Could you check a few things on this drawing? It's one solid part, dimensions in mm from its lowest x, y, z. A direction names the side the tool comes from. Round coordinates to 2 decimals unless told otherwise and drop trailing zeros. Write each loop counter-clockwise with the first axis right and the second up, starting at its lowest first coordinate (ties: lowest second). Pieces come first, ordered by that corner, then holes. Notation, with made-up numbers: (-38.5, 60.5) - (-17.5, 60.5) arc R3 cw to (-17.5, 65.5) - close; hole circle Ø4 at (-35.75, 81). An arc over 180 degrees is marked (long way). Use one line per item in the form item = value. Start each with the question number.
1. I want a section at C-C, the plane z = 17.5. List the corners of the cut face in (x, y) for me.
2. I want a section at B-B, the plane x = 5. List the corners of the cut face in (y, z) for me, plus the area to 3 significant figures.
3. Which directions (+Z, -Z, +X, -X, +Y, -Y) give clear straight access to the entire face, cutting with the end or side of a thin tool? Please do the marked faces 5, 6, 7 and 8.
4. If I drill on line 1 along X through (y, z) = (8.75, 17); line 2 along Y through (x, z) = (1.5, 9); line 3 along X through (y, z) = (17.5, 19), over which ranges is the centre line in solid material (lowest first)?
5. I want a section at A-A, the plane y = 4.75. List the corners of the cut face in (x, z) for me.
6. Will these pins go through, and if not, where does the flat tip stop? pin 1 (3 mm diameter, centred on y = 14.5, z = 19, fed in from +X); pin 2 (4 mm diameter, centred on x = 7.5, z = 19, fed in from -Y); pin 3 (5 mm diameter, centred on x = 16, z = 16.5, fed in from +Y); pin 4 (3 mm diameter, centred on x = 13.5, y = 1.5, fed in from -Z).
7. We'd pull the mould along Z, two halves only. Please class the marked faces 1, 2, 3 and 4: +Z half, -Z half, draft (parallel to the pull), parting line (faces both ways), or undercut.
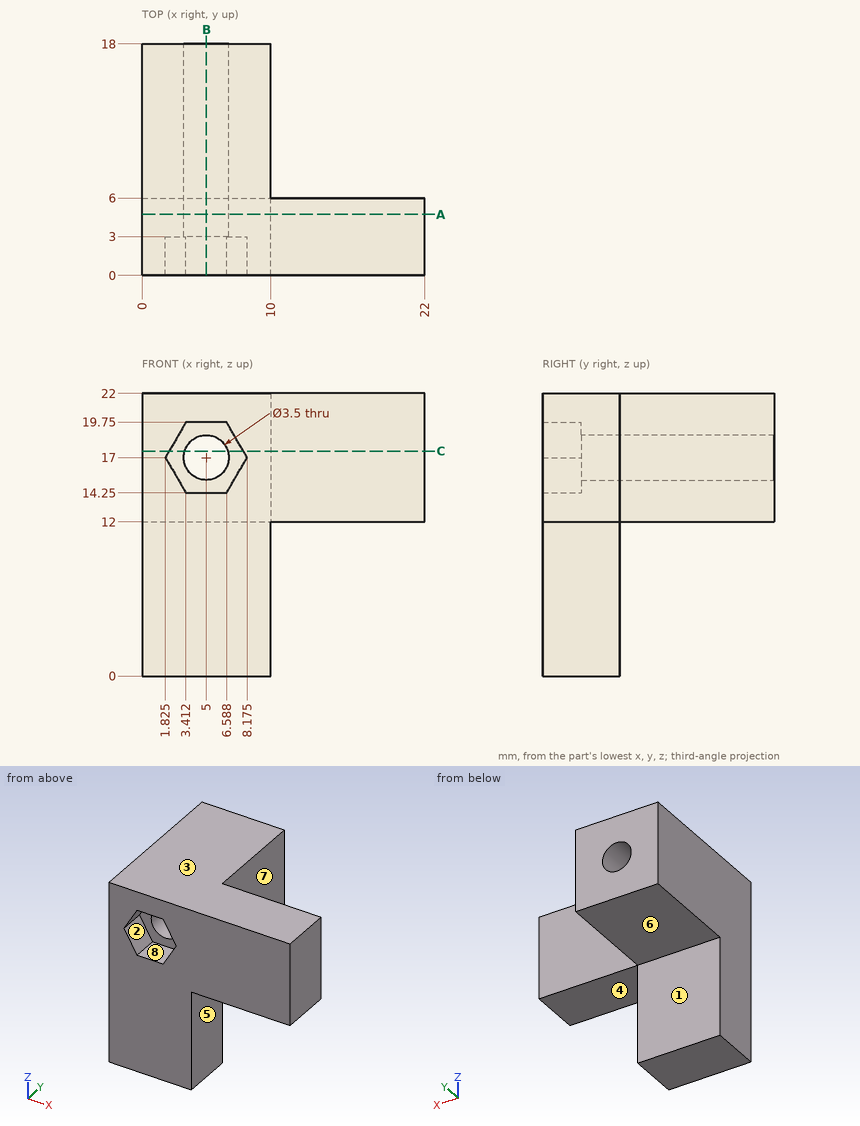
Model answer:
q1.outline = (0, 0) - (2.11, 0) - (2.11, 3) - (3.32, 3) - (3.32, 18) - (0, 18) - close; (6.68, 3) - (7.89, 3) - (7.89, 0) - (22, 0) - (22, 6) - (10, 6) - (10, 18) - (6.68, 18) - close
q2.outline = (0, 0) - (6, 0) - (6, 12) - (18, 12) - (18, 15.25) - (3, 15.25) - (3, 14.25) - (0, 14.25) - close; (0, 19.75) - (3, 19.75) - (3, 18.75) - (18, 18.75) - (18, 22) - (0, 22) - close
q2.area = 183 mm2
q3.face_5 = -Z, +X, +Y, -Y
q3.face_6 = -Z, +X, -X, +Y
q3.face_7 = +Z, -Z, +X, +Y
q3.face_8 = -Y
q4.line_1 = 0 to 3.25, 6.75 to 10
q4.line_2 = 0 to 6
q4.line_3 = 0 to 10
q5.outline = (0, 0) - (10, 0) - (10, 12) - (22, 12) - (22, 22) - (0, 22) - close; hole circle Ø3.5 at (5, 17)
q6.pin_1 = 10
q6.pin_2 = 0
q6.pin_3 = 6
q6.pin_4 = 12
q7.face_1 = draft
q7.face_2 = undercut
q7.face_3 = +Z half
q7.face_4 = -Z half
